Can you work these out from the model? Positions are in its coordinate system, mm. Give positions to 0.01 mm unless a question says otherwise; leave off trailing zeros. Write each loop counter-clockwise with the first axis right and the second up, starting at its lowest first coordinate (ties: lowest second). Pieces come first, ordered by that corner, then holes. Notation, with made-up numbers: M -12.5,70 L 15.5,70 A20 cw 15.5,77 Z; hole C 34,23.25 d8. An arc over 180 degrees is marked long. Use CSV: the item, a comma, the result in double quotes. Start each with the question number.
from build123d import *

# Parameters (mm, degrees)
SKETCH1_R           = 3.5
BOSS_EXTRUDE1_DEPTH = 10
BOSS_EXTRUDE2_START = 2
SKETCH2_R           = 1
BOSS_EXTRUDE2_DEPTH = 2


with BuildPart() as part:
    # Sketch1 → Boss-Extrude1 (new body)
    with BuildSketch(Plane.XY):
        Circle(SKETCH1_R)
    extrude(amount=BOSS_EXTRUDE1_DEPTH)

    # Sketch2 → Boss-Extrude2 (add)
    with BuildSketch(Plane(origin=(0, 0, 0), x_dir=(-1, 0, 0), z_dir=(0, 0, -1)).offset(BOSS_EXTRUDE2_START)):
        with BuildLine():
            Line((-3.5, 0), (-3.5, 30))
            Line((-3.5, 30), (3.5, 30))
            Line((3.5, 30), (3.5, 0))
            ThreePointArc((3.5, 0), (0, -3.5), (-3.5, 0))
        make_face()
        with Locations((0, 27)):
            Circle(SKETCH2_R, mode=Mode.SUBTRACT)
    extrude(amount=-BOSS_EXTRUDE2_DEPTH)


solid = part.part
(1) Thinking about a two-plate mould opening in Y: for faces 1 (the face through (-3.5, 15, -1)), 2 (the face through (0, 30, -1)), 3 (the face through (0, 28, -1)), which applies, released by +Y, released by -Y, zero draft, split by the parting line, or undercut?
(2) I want a section at D-D (y = 21.5). Write out the boundary of the cut face in (x, z), and give its area (3 significant figures).
(3) I want a section at A-A (x = 0). Write out the boundary of the cut face in (y, z), and give its area (3 significant figures).
(4) Will these pins go through, and if not, where does the flat tip stop? pin 1 Ø1 at (x, z) = (0.5, 7) entering from -Y; pin 2 Ø2 at (x, y) = (1.5, 10.5) entering from +Z.
(5) Please list where these lines run through material, in increasing order: L1, parallel to Y at x = 0, z = -1.45; L2, parallel to Z at x = -0.5, y = 16.5; L3, parallel to Y at x = 0, z = 2.25. Write a range as [from, to].
(6) I want a section at C-C (z = 3.75). Write out the boundary of the cut face in (x, y), and give its area (3 significant figures).
(7) I want a section at B-B (y = 27). Write out the boundary of the cut face in (x, z).
Geometry results:
1,face 1,"zero draft"
1,face 2,"released by +Y"
1,face 3,"undercut"
2,outline,"M -3.5,-2 L 3.5,-2 L 3.5,0 L -3.5,0 Z"
2,area,"14.0 mm2"
3,outline,"M -3.5,-2 L 26,-2 L 26,0 L 3.5,0 L 3.5,10 L -3.5,10 Z; M 28,-2 L 30,-2 L 30,0 L 28,0 Z"
3,area,"133 mm2"
4,pin 1,"stops at y = -3.5"
4,pin 2,"stops at z = 0"
5,L1,"y = [-3.5, 26], [28, 30]"
5,L2,"z = [-2, 0]"
5,L3,"y = [-3.5, 3.5]"
6,outline,"C 0,0 d7"
6,area,"38.5 mm2"
7,outline,"M -3.5,-2 L -1,-2 L -1,0 L -3.5,0 Z; M 1,-2 L 3.5,-2 L 3.5,0 L 1,0 Z"
